Check sheet for the modelled part. Datum: model origin and axes. Units: mm. A direction names the side the tool comes from. Give positions to 0.01 mm unless a question says otherwise; leave off trailing zeros. Loops run counter-clockwise (first coordinate to the right, second up) from the corner with the lowest first, then second, coordinate; pieces in that order, holes last. Notation, with made-up numbers: (37.5, 62) -> (58.5, 62) arc R30 cw to (58.5, 92) -> close; hole circle Ø11 at (20.25, 87). An arc over 180 degrees is marked (long way). Write each question's results on one line, items separated by ' | '. Start each with the question number.
1. Gauge pin test, flat end, axial feed: pin 1 Ø3 at (x, y) = (40.5, -24) entering from -Z. Record the tip position at first contact, or that the pin passes through.
2. Tool access check on faces 1 (the face through (16, -47.494, -6)), 2 (the face through (50.84, 4.65, -7.6)). Record the directions out of +Z, -Z, +X, -X, +Y, -Y that give a thin tool (end or side, any length) a straight path to the whole face; none if there is none.
3. Cross-section at B-B on x = 30. Record the boundary of the cut face in (y, z).
4. Material ranges on L1, parallel to X at y = -5, z = -0.25; L2, parallel to Y at x = 43, z = -2; L3, parallel to Z at x = 8, y = -38, recorded low to high. Write a range as from..to.
5. Cross-section at A-A on z = -5.75. Record the boundary of the cut face in (x, y), and give its area (3 significant figures).
6. Cross-section at C-C on y = -22. Record the boundary of the cut face in (x, z), and give its area (3 significant figures).
7. Mould release check, pull along Y, two halves, no side actions. Record for faces 3 (the face through (54.741, -20, -6)), 4 (the face through (51.741, -19, -7)), 5 (the face through (17, 8.506, -6)): +Y half, -Y half, draft (parallel to the pull), parting line (faces both ways), or undercut.
Autodesk Inventor part; units mm, degrees
ref_plane "YZ Plane" through (0, 0, 0) normal (1, 0, 0) x (0, 1, 0)
ref_plane "XZ Plane" through (0, 0, 0) normal (0, 1, 0) x (-1, 0, 0)
ref_plane "XY Plane" through (0, 0, 0) normal (0, 0, 1) x (1, 0, 0)
sketch "Sketch1" plane through (0, 0, 0) normal (0, 0, 1) x (1, 0, 0)
  line L0 (-18.2588, 5.5059) -> (51.7412, 5.5059)
  line L1 (51.7412, 5.5059) -> (51.7412, -44.4941)
  line L2 (51.7412, -44.4941) -> (-18.2588, -44.4941)
  line L3 (-18.2588, -44.4941) -> (-18.2588, 5.5059)
  line L4 (54.7412, 8.5059) -> (-21.2588, 8.5059)
  line L5 (-21.2588, 8.5059) -> (-21.2588, -47.4941)
  line L6 (-21.2588, -47.4941) -> (54.7412, -47.4941)
  line L7 (54.7412, -47.4941) -> (54.7412, 8.5059)
  point P0 (0, 0)
  dimension "d0" = 70
  dimension "d1" = 50
  dimension "d2" = 3
extrude "Extrusion1" add sketch "Sketch1" along normal blind 3 contours L0 L1 L2 L3 | L7 L6 L5 L4
extrude "Extrusion2" add sketch "Sketch1" against normal blind 15
fillet "Fillet1" radius 3 8 edges at (51.7412, -44.4941, -7.5) (54.7412, -47.4941, -6) (54.7412, 8.5059, -6) (51.7412, 5.5059, -7.5) (-21.2588, 8.5059, -6) (-18.2588, 5.5059, -7.5) (-18.2588, -44.4941, -7.5) (-21.2588, -47.4941, -6)
properties part number "3DP_PLA_Tray_for_unknown_parts" material "ABS Plastic"
Geometry says:
1) pin 1: z = 0
2) face 1: +Z, -Z, +X, -X, -Y | face 2: -Z
3) outline: (-47.49, -15) -> (-44.49, -15) -> (-44.49, 0) -> (5.51, 0) -> (5.51, -15) -> (8.51, -15) -> (8.51, 3) -> (-47.49, 3) -> close
4) L1: -21.26..-18.26, 51.74..54.74 | L2: -47.49..-44.49, 5.51..8.51 | L3: 0..3
5) outline: (-21.26, -44.49) arc R3 ccw to (-18.26, -47.49) -> (51.74, -47.49) arc R3 ccw to (54.74, -44.49) -> (54.74, 5.51) arc R3 ccw to (51.74, 8.51) -> (-18.26, 8.51) arc R3 ccw to (-21.26, 5.51) -> close; hole (-18.26, -41.49) arc R3 ccw to (-15.26, -44.49) -> (48.74, -44.49) arc R3 ccw to (51.74, -41.49) -> (51.74, 2.51) arc R3 ccw to (48.74, 5.51) -> (-15.26, 5.51) arc R3 ccw to (-18.26, 2.51) -> close | area: 756 mm^2
6) outline: (-21.26, -15) -> (-18.26, -15) -> (-18.26, 0) -> (51.74, 0) -> (51.74, -15) -> (54.74, -15) -> (54.74, 3) -> (-21.26, 3) -> close | area: 318 mm^2
7) face 3: draft | face 4: undercut | face 5: +Y half
